```python
from build123d import *

# Parameters (mm, degrees)
PAD027_DEPTH    = 2
PAD028_DEPTH    = 25
PAD029_DEPTH    = 33
SKETCH050_R     = 1.5
SKETCH050_R_2   = 5
POCKET020_DEPTH = 101.5
SKETCH051_W     = 50
SKETCH051_H     = 37
SKETCH051_W_2   = 42
SKETCH051_H_2   = 29
PAD030_DEPTH    = 10
POCKET021_DEPTH = 63.5


with BuildPart() as part:
    # Sketch046 → Pad027 (new body)
    with BuildSketch(Plane.XY):
        Polygon((16.5, 65.5), (-16.5, 88.5), (-66.5, 88.5), (-80, 51.5), (-80, -51.5), (-16.5, -51.5), (-16.5, -65.5), (16.5, -88.5), (66.5, -88.5), (80, -51.5), (80, 51.5), (16.5, 51.5), align=None)
    extrude(amount=-PAD027_DEPTH)

    # Sketch047 → Pad028 (join)
    with BuildSketch(Plane.XY):
        Polygon((76, 47.5), (76, -47.5), (15.5, -47.5), (-15.5, -47.5), (-76, -47.5), (-76, 47.5), (-15.5, 47.5), (15.5, 47.5), (36, 47.5), (36, 51.5), (15.5, 51.5), (-15.5, 51.5), (-80, 51.5), (-80, -51.5), (-15.5, -51.5), (15.5, -51.5), (80, -51.5), (80, 51.5), (66, 51.5), (66, 47.5), align=None)
    extrude(amount=PAD028_DEPTH)

    # Sketch048 (on Face7 of Pad028) → Pad029 (join)
    with BuildSketch(Plane.XY):
        Polygon((-16.5, 67.5), (16.5, 67.5), (16.5, 51.5), (16.5, 47.5), (-16.5, 47.5), (-16.5, 51.5), align=None)
        Polygon((16.5, -51.5), (16.5, -67.5), (-16.5, -67.5), (-16.5, -51.5), (-16.5, -47.5), (16.5, -47.5), align=None)
    extrude(amount=PAD029_DEPTH)

    # Sketch050 → Pocket020 (cut, symmetric)
    with BuildSketch(Plane.XZ):
        with Locations((-12.020815, 4.479185)):
            Circle(SKETCH050_R)
        with Locations((12.020815, 28.520815)):
            Circle(SKETCH050_R)
        with Locations((-12.020815, 28.520815)):
            Circle(SKETCH050_R)
        with Locations((12.020815, 4.479185)):
            Circle(SKETCH050_R)
        with Locations((0, 16.5)):
            Circle(SKETCH050_R_2)
    extrude(amount=POCKET020_DEPTH, both=True, mode=Mode.SUBTRACT)

    # Sketch051 → Pad030 (join)
    with BuildSketch(Plane.XY):
        with Locations((-41.5, 70)):
            Rectangle(SKETCH051_W, SKETCH051_H)
        with Locations((-41.5, 70)):
            Rectangle(SKETCH051_W_2, SKETCH051_H_2, mode=Mode.SUBTRACT)
        with Locations((41.5, -70)):
            Rectangle(SKETCH051_W, SKETCH051_H)
        with Locations((41.5, -70)):
            Rectangle(SKETCH051_W_2, SKETCH051_H_2, mode=Mode.SUBTRACT)
    extrude(amount=PAD030_DEPTH)

    # Sketch058 → Pocket021 (cut, symmetric)
    with BuildSketch(Plane.XZ):
        with BuildLine():
            Line((-16.5, 33), (-16.5, 24.041631))
            ThreePointArc((-16.5, 24.041631), (-7.541631, 24.041631), (-7.541631, 33))
            Line((-16.5, 33), (-7.541631, 33))
        make_face()
        with BuildLine():
            Line((16.5, 33), (16.5, 24.041631))
            ThreePointArc((7.541631, 33), (7.541631, 24.041631), (16.5, 24.041631))
            Line((16.5, 33), (7.541631, 33))
        make_face()
        with BuildLine():
            Line((-16.5, 0), (-16.5, 8.958369))
            ThreePointArc((-7.541631, 0), (-7.541631, 8.958369), (-16.5, 8.958369))
            Line((-16.5, 0), (-7.541631, 0))
        make_face()
        with BuildLine():
            Line((16.5, 0), (7.541631, 0))
            ThreePointArc((16.5, 8.958369), (7.541631, 8.958369), (7.541631, 0))
            Line((16.5, 0), (16.5, 8.958369))
        make_face()
    extrude(amount=POCKET021_DEPTH, both=True, mode=Mode.SUBTRACT)


solid = part.part
```
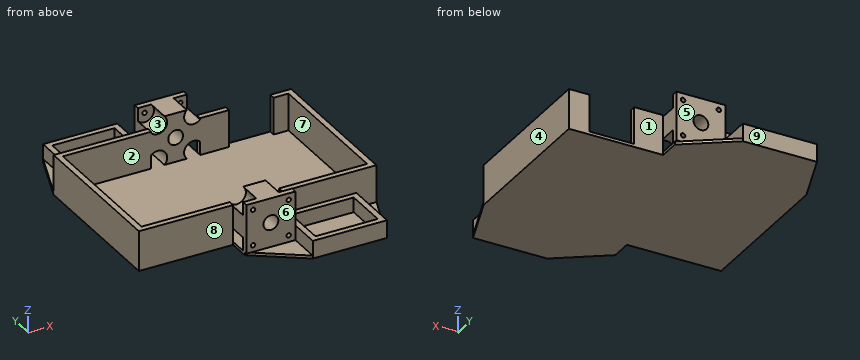
CAD build for the part. Positions are in the model's coordinates, mm. Face numbers are marked on the shaded views. A direction names the side the tool comes from. Coordinates: 2 decimals unless noted, no trailing zeros. Loops run counter-clockwise (first coordinate to the right, second up) from the corner with the lowest first, then second, coordinate; pieces in that order, holes last. Notation, with made-up numbers: (69.25, -11.75) - (77.25, -11.75) arc R30 cw to (77.25, 23.25) - close; hole circle Ø5 at (44, 29.25). An arc over 180 degrees is marked (long way). Return JSON: item names as keys, results as strings.
1. Drop flat-ended pins along their axis: pin 1 (5.5 mm diameter, centred on x = 11, z = 29.5, fed in from -Y); pin 2 (1.5 mm diameter, centred on x = -10, y = 31.5, fed in from +Z); pin 3 (4 mm diameter, centred on x = 34.5, z = 19, fed in from +Y). Give the stop position or say it passes through.
Result:
{"pin 1": "stops at y = -67.5", "pin 2": "stops at z = 0", "pin 3": "stops at y = 51.5"}
2. Probe L1, parallel to Y at x = -46, z = 6.5; L2, parallel to Y at x = -8, z = 5.5; L3, parallel to Y at x = 24.5, z = 5. List the from-to ranges inside material, lowest first. Write a range as from..to.
Result:
{"L1": "y = -51.5..-47.5, 47.5..55.5, 84.5..88.5", "L2": "y = -67.5..-63.5, 63.5..67.5", "L3": "y = -88.5..-84.5, -55.5..-47.5, 47.5..51.5"}
3. Band-saw the part on C-C (y = -35.5). Give the cut face in (x, z), and give its area (3 significant figures).
Result:
{"outline": "(-80, -2) - (80, -2) - (80, 25) - (76, 25) - (76, 0) - (-76, 0) - (-76, 25) - (-80, 25) - close", "area": "520 mm2"}
4. Band-saw the part on A-A (z = 16.5). Give the cut face in (x, y).
Result:
{"outline": "(-80, -51.5) - (-16.5, -51.5) - (-16.5, -67.5) - (-5, -67.5) - (-5, -47.5) - (-76, -47.5) - (-76, 47.5) - (-5, 47.5) - (-5, 67.5) - (-16.5, 67.5) - (-16.5, 51.5) - (-80, 51.5) - close; (5, -67.5) - (16.5, -67.5) - (16.5, -51.5) - (80, -51.5) - (80, 51.5) - (66, 51.5) - (66, 47.5) - (76, 47.5) - (76, -47.5) - (5, -47.5) - close; (5, 47.5) - (36, 47.5) - (36, 51.5) - (16.5, 51.5) - (16.5, 67.5) - (5, 67.5) - close"}
5. Band-saw the part on B-B (x = 0). Give the cut face in (y, z).
Result:
{"outline": "(-77, -2) - (77, -2) - (77, 0) - (67.5, 0) - (67.5, 11.5) - (47.5, 11.5) - (47.5, 0) - (-47.5, 0) - (-47.5, 11.5) - (-67.5, 11.5) - (-67.5, 0) - (-77, 0) - close; (-67.5, 21.5) - (-47.5, 21.5) - (-47.5, 33) - (-67.5, 33) - close; (47.5, 21.5) - (67.5, 21.5) - (67.5, 33) - (47.5, 33) - close"}
6. Band-saw the part on D-D (x = 23). Give the cut face in (y, z).
Result:
{"outline": "(-88.5, -2) - (51.5, -2) - (51.5, 25) - (47.5, 25) - (47.5, 0) - (-47.5, 0) - (-47.5, 25) - (-51.5, 25) - (-51.5, 10) - (-55.5, 10) - (-55.5, 0) - (-84.5, 0) - (-84.5, 10) - (-88.5, 10) - close"}
7. Mould opens along Y. For the marked faces 1, 2, 3 and 4 say: released by +Y, released by -Y, zero draft, split by the parting line, or undercut.
Result:
{"face 1": "released by +Y", "face 2": "undercut", "face 3": "undercut", "face 4": "zero draft"}
8. 3-axis set-ups, long thin cutter, end or side, ignore diameter. For the marked faces 5, 6, 7, 8 and 9: which of +Z, -Z, +X, -X, +Y, -Y reach the whole face in a straight line?
Result:
{"face 5": "+Z, +X, +Y", "face 6": "+Z, -X, -Y", "face 7": "+Z", "face 8": "+Z, -Z, -X, -Y", "face 9": "+Z, -Z, +X, -X, +Y"}
